The figure shows three views and two pictorial views of one solid part (mm, origin at its lowest corner). Answer the questions. A direction names the side the tool comes from. Coordinates: 2 decimals unless noted, no trailing zeros. Loops run counter-clockwise (first coordinate to the right, second up) from the corner with the lowest first, then second, coordinate; pieces in that order, holes last. Notation, with made-up numbers: M -32.75,9 L 19.25,9 A14 ccw 19.25,15 Z; hole C -22.5,45.25 d11. An arc over 180 degrees is marked long. Write each question's results on one line, items separated by ' | '.
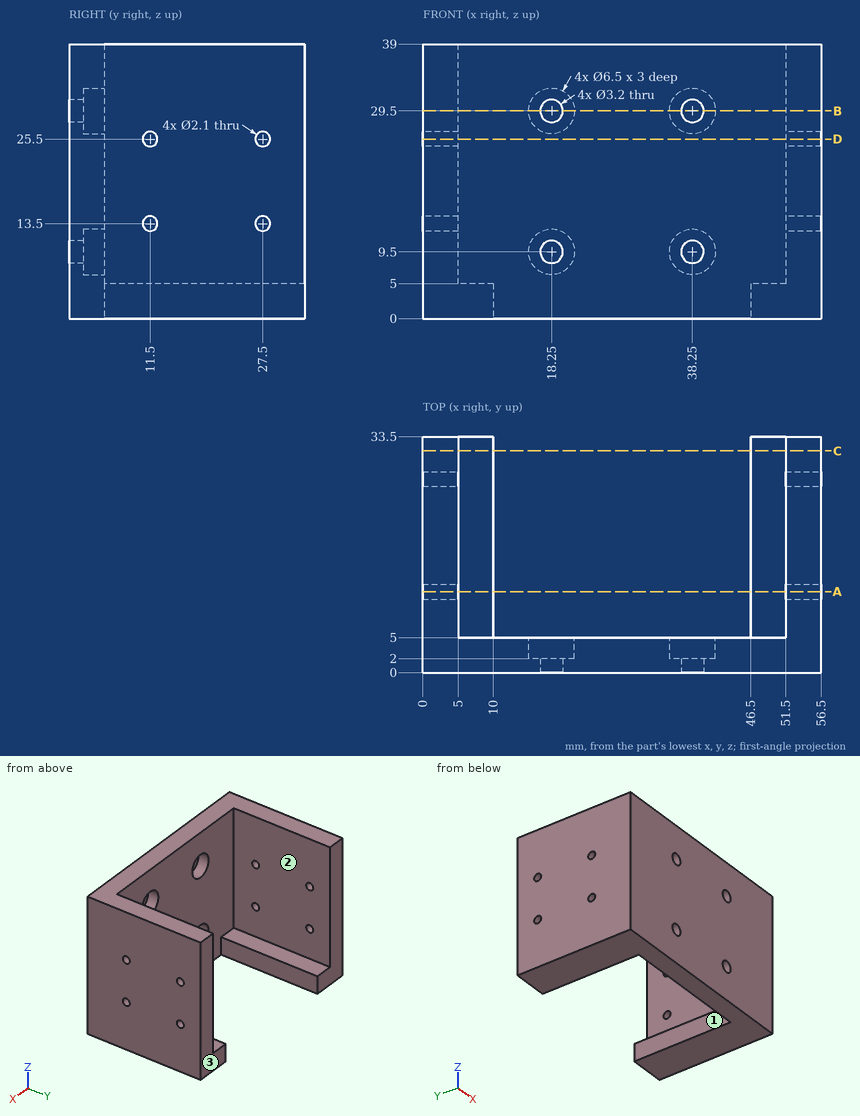
1) Which of the six approach directions +Z, -Z, +X, -X, +Y, -Y give full straight-line access (tool end or side, diameter ignored) to the marked faces 1, 2 and 3?
Check result:
face 1: +Z, -Z, +Y | face 2: +Z, +Y | face 3: +Z, -Z, +X, -X, +Y
2) Find section C-C, the plane y = 31.5. Give the vertices of the cut face in (x, z), and give its area (3 significant figures).
Check result:
outline: M 0,0 L 10,0 L 10,5 L 5,5 L 5,39 L 0,39 Z; M 46.5,0 L 56.5,0 L 56.5,39 L 51.5,39 L 51.5,5 L 46.5,5 Z | area: 440 mm^2
3) Given pin 1 Ø3 at (x, z) = (15.5, 12) entering from +Y; pin 2 Ø12 at (x, y) = (43, 26) entering from +Z, each flat-ended and moving along its own axis, determine where each tip first touches the part or whether it passes through.
Check result:
pin 1: y = 5 | pin 2: z = 5
4) Find section A-A, the plane y = 11.5. Give the vertices of the cut face in (x, z).
Check result:
outline: M 0,0 L 10,0 L 10,5 L 5,5 L 5,12.45 L 0,12.45 Z; M 0,14.55 L 5,14.55 L 5,24.45 L 0,24.45 Z; M 0,26.55 L 5,26.55 L 5,39 L 0,39 Z; M 46.5,0 L 56.5,0 L 56.5,12.45 L 51.5,12.45 L 51.5,5 L 46.5,5 Z; M 51.5,14.55 L 56.5,14.55 L 56.5,24.45 L 51.5,24.45 Z; M 51.5,26.55 L 56.5,26.55 L 56.5,39 L 51.5,39 Z
5) Find section D-D, the plane z = 25.5. Give the vertices of the cut face in (x, y), and give its area (4 significant figures).
Check result:
outline: M 0,0 L 56.5,0 L 56.5,10.45 L 51.5,10.45 L 51.5,5 L 5,5 L 5,10.45 L 0,10.45 Z; M 0,12.55 L 5,12.55 L 5,26.45 L 0,26.45 Z; M 0,28.55 L 5,28.55 L 5,33.5 L 0,33.5 Z; M 51.5,12.55 L 56.5,12.55 L 56.5,26.45 L 51.5,26.45 Z; M 51.5,28.55 L 56.5,28.55 L 56.5,33.5 L 51.5,33.5 Z | area: 525.5 mm^2
6) Straight lines are drawn through the part: probe 1 along X at (y, z) = (12.5, 29); probe 2 along X at (y, z) = (22.5, 2); probe 3 along Z at (x, y) = (18, 1). For each, find the intervals that lie inside material, in ascending order. Write a range as [from, to].
Check result:
probe 1: [0, 5], [51.5, 56.5] | probe 2: [0, 10], [46.5, 56.5] | probe 3: [0, 7.92], [11.08, 27.92], [31.08, 39]
7) Find section B-B, the plane z = 29.5. Give the vertices of the cut face in (x, y).
Check result:
outline: M 0,0 L 16.65,0 L 16.65,2 L 15,2 L 15,5 L 5,5 L 5,33.5 L 0,33.5 Z; M 19.85,0 L 36.65,0 L 36.65,2 L 35,2 L 35,5 L 21.5,5 L 21.5,2 L 19.85,2 Z; M 39.85,0 L 56.5,0 L 56.5,33.5 L 51.5,33.5 L 51.5,5 L 41.5,5 L 41.5,2 L 39.85,2 Z
